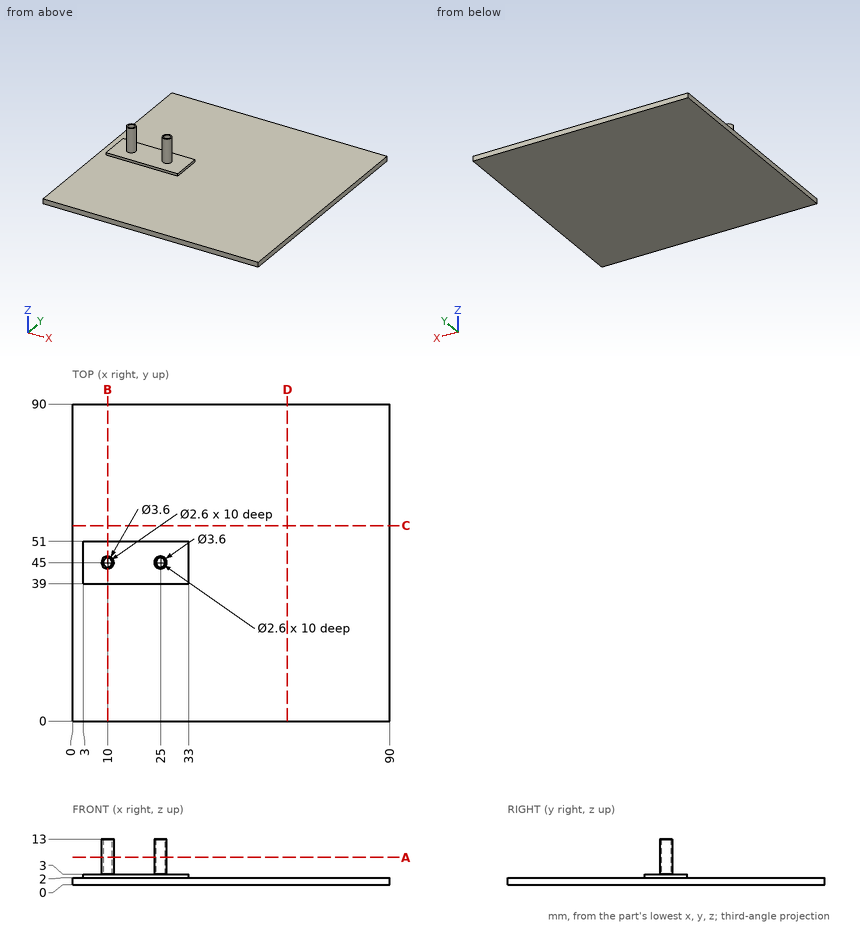
Can you work these out from the drawing? Everything is in mm from the part's minimum corner. Coordinates: 2 decimals unless noted, no trailing zeros. Write each loop counter-clockwise with the first axis right and the second up, starting at its lowest first coordinate (ties: lowest second). Pieces come first, ordered by that corner, then holes. Notation, with made-up numbers: (65, 29) - (111, 29) arc R12 cw to (111, 41) - close; hole circle Ø1 at (23.25, 77). An arc over 180 degrees is marked (long way). One line per item, written item: value.
1) Suppose I cut it at C-C on y = 55.5. Write out the boundary of the cut face in (x, z), and give its area (3 significant figures).
Model answer:
outline: (0, 0) - (90, 0) - (90, 2) - (0, 2) - close
area: 180 mm²
2) Suppose I cut it at B-B on x = 10. Write out the boundary of the cut face in (y, z).
Model answer:
outline: (0, 0) - (90, 0) - (90, 2) - (51, 2) - (51, 3) - (46.8, 3) - (46.8, 13) - (46.3, 13) - (46.3, 3) - (43.7, 3) - (43.7, 13) - (43.2, 13) - (43.2, 3) - (39, 3) - (39, 2) - (0, 2) - close
3) Suppose I cut it at A-A on z = 7.75. Write out the boundary of the cut face in (x, y).
Model answer:
outline: circle Ø3.6 at (10, 45); circle Ø3.6 at (25, 45); hole circle Ø2.6 at (10, 45); hole circle Ø2.6 at (25, 45)
4) I'm going to push flat-ended pins straight in: P1, Ø2, axis at x = 61, y = 59.5, coming from the +Z side; P2, Ø1.5, axis at y = 28, z = 4, coming from the +X side; P3, Ø0.8, axis at x = 17.5, z = 2.5, coming from the +Y side; P4, Ø1.3, axis at x = 25, y = 44.5, coming from the +Z side. Where does each tip first touch, or does it pass through?
Model answer:
P1: stops at z = 2
P2: passes through
P3: stops at y = 51
P4: stops at z = 3
5) I need wall thicknesses on line 1 along Y through (x, z) = (25, 11.25); line 2 along Z through (x, y) = (51, 46); line 3 along Z through (x, y) = (10, 47). Which ranges of each line are inside material? Lowest first, please.
Model answer:
line 1: y = 43.2 to 43.7, 46.3 to 46.8
line 2: z = 0 to 2
line 3: z = 0 to 3
